Verification items for the finished model (mm, model axes). Round coordinates to 2 decimals unless told otherwise and drop trailing zeros. Write each loop counter-clockwise with the first axis right and the second up, starting at its lowest first coordinate (ties: lowest second). Pieces come first, ordered by that corner, then holes. Notation, with made-up numbers: M 10,20 L 42,20 A32 ccw 42,53 Z; hole C -29.75,-6 d7. An arc over 180 degrees is marked long. One line per item, written item: value. Start each with the question number.
Autodesk Inventor part; units mm, degrees
ref_plane "YZ Plane" through (0, 0, 0) normal (1, 0, 0) x (0, 1, 0)
ref_plane "XZ Plane" through (0, 0, 0) normal (0, 1, 0) x (-1, 0, 0)
ref_plane "XY Plane" through (0, 0, 0) normal (0, 0, 1) x (1, 0, 0)
sketch "Sketch1" plane through (0, 0, 0) normal (0, 0, 1) x (1, 0, 0)
  line L0 (0, 14) -> (0, -14)
  line L1 (-33.3375, 0) -> (33.3375, 0)
  line L2 (23.8125, -10) -> (-23.8125, -10)
  line L3 (-23.8125, -10) -> (-23.8125, 10)
  line L4 (-23.8125, 10) -> (23.8125, 10)
  line L5 (23.8125, 10) -> (23.8125, -10)
  line L6 (23.8125, -10) -> (-23.8125, 10) construction
  line L7 (-23.8125, -10) -> (23.8125, 10) construction
  point P0 (0, 0)
  point P1 (-14, 0)
  point P2 (14, 0)
  dimension "d0" = 47.625
  dimension "d1" = 14
  dimension "d2" = 14
  dimension "d3" = 20
extrude "Extrusion1" add sketch "Sketch1" along normal blind 6.35
hole "Hole1" at (-14, 0, 0) at (14, 0, 0) direction (0, 0, 1) diameter 6.985 end through all
fillet "Fillet1" radius 3.175 4 edges at (23.8125, 10, 3.175) (23.8125, -10, 3.175) (-23.8125, -10, 3.175) (-23.8125, 10, 3.175)
1) Thickness scan on line 1 (X direction, y = 0, z = 2.5); line 2 (Y direction, x = -14, z = 5); line 3 (X direction, y = -2, z = 3). Record the ranges inside material, lowest first.
2) Cross-section at B-B (y = 0). Record the boundary of the cut face in (x, z).
3) Cross-section at D-D (x = -17). Record the boundary of the cut face in (y, z).
4) Mould release check, pull along Y, two halves, no side actions. Record for faces 1 (the flat face through (0, 0, 6.35)), 2 (the cylindrical face through (17.4, -0.8, 3.2)), 3 (the cylindrical face through (-22.86, 9.09, 3.22)): pulls with the +Y half, pulls with the -Y half, needs draft (parallel to the pull), parting line crosses it, or undercut.
5) Cross-section at A-A (x = 14). Record the boundary of the cut face in (y, z).
6) Cross-section at C-C (z = 1.25). State how many separate pieces and enclosed holes the cut face has, then the cut area to 3 significant figures.
7) Gauge pin test, flat end, axial feed: pin 1 Ø6.5 at (x, y) = (14, 0) entering from -Z. Record the tip position at first contact, or that the pin passes through.
Results below:
1. line 1: x = -23.81 to -17.49, -10.51 to 10.51, 17.49 to 23.81
1. line 2: y = -10 to -3.49, 3.49 to 10
1. line 3: x = -23.81 to -16.86, -11.14 to 11.14, 16.86 to 23.81
2. outline: M -23.81,0 L -17.49,0 L -17.49,6.35 L -23.81,6.35 Z; M -10.51,0 L 10.51,0 L 10.51,6.35 L -10.51,6.35 Z; M 17.49,0 L 23.81,0 L 23.81,6.35 L 17.49,6.35 Z
3. outline: M -10,0 L -1.79,0 L -1.79,6.35 L -10,6.35 Z; M 1.79,0 L 10,0 L 10,6.35 L 1.79,6.35 Z
4. face 1: needs draft
4. face 2: undercut
4. face 3: pulls with the +Y half
5. outline: M -10,0 L -3.49,0 L -3.49,6.35 L -10,6.35 Z; M 3.49,0 L 10,0 L 10,6.35 L 3.49,6.35 Z
6. separate pieces: 1
6. enclosed holes: 2
6. area: 867 mm²
7. pin 1: passes through
